Could you check a few things on this model? Use its own coordinates, in mm. A direction names the side the tool comes from. Coordinates: 2 decimals unless noted, no trailing zeros. Write each loop counter-clockwise with the first axis right and the second up, starting at its lowest first coordinate (ties: lowest second). Pieces come first, ordered by that corner, then holes.
Item 1: Which directions (+Z, -Z, +X, -X, +Y, -Y) give clear straight access to the entire face, cutting with the end or side of a thin tool? Please do faces 4 (the cylindrical face through (-16.52, -108.6, 7.96)), 5 (the flat face through (-18, 69, 7)), 6 (the flat face through (-25.2, 0.6, 13.75)), 7 (the flat face through (-18, -68, 7)).
Item 2: Thinking about a two-plate mould opening in Z: for faces 1 (the cylindrical face through (-16.52, 82.6, 7.96)), 2 (the flat face through (-22.4, 1.7, 15.75)), 3 (the cylindrical face through (-27, 0, 15)), which applies, +Z half, -Z half, draft (parallel to the pull), parting line (faces both ways), or undercut?
Item 3: I want a section at B-B on z = 2. Please give me the cut outline in (x, y).
Item 4: I want a section at C-C on y = -28. Please give me the cut outline in (x, z).
Item 5: If I drill on probe 1 along Z at (x, y) = (-16.75, -62.8) (3 decimals); probe 2 along X at (y, z) = (24, 11.5); probe 3 along Z at (x, y) = (-19, 22), over which ranges is the centre line in solid material (lowest first)?
Item 6: I want a section at D-D on y = 5. Please give me the cut outline in (x, z).
Item 7: For P1, Ø4.5, axis at y = 80.6, z = 7.875, coming from the -X side; P2, Ø3, axis at y = 32.8, z = 7.875, coming from the +X side; P3, Ø1, axis at y = -91, z = 14.5, coming from the -X side; P4, Ø2.5, axis at x = -21, y = 43.5, coming from the -Z side, each with a flat end and sliding along its axis, tell me the tip position at first contact or that it passes through.
Item 8: I want a section at A-A on y = 62.8. Please give me the cut outline in (x, z) (3 decimals), then the cut area to 4 significant figures.
from build123d import *

# Parameters (mm, degrees)
F1_DEPTH = 15.75
F2_R     = 2
F4_DEPTH = 3.001
F3_R     = 2
F5_DEPTH = 3.001
F7_DEPTH = 2


# Not quite as in the source:
# - a feature names something its author has since deleted; it is built from what else it names


with BuildPart() as f1:
    # F0 (on Top) → F1 (new body)
    with BuildSketch(Plane.XY):
        with BuildLine():
            Line((-15, 119.5), (-18, 119.5))
            Line((-18, 119.5), (-18, 17.3493515729))
            ThreePointArc((-18, 17.3493515729), (-25, 0), (-18, -17.3493515729))
            Line((-18, -17.3493515729), (-18, -119.5))
            Line((-18, -119.5), (-15, -119.5))
            Line((-15, -119.5), (-15, -16.0934769394))
            ThreePointArc((-15, -16.0934769394), (-16.5896327506, -14.4493627956), (-18, -12.6491106407))
            ThreePointArc((-18, -12.6491106407), (-22, 0), (-18, 12.6491106407))
            ThreePointArc((-18, 12.6491106407), (-16.5896327506, 14.4493627956), (-15, 16.0934769394))
            Line((-15, 16.0934769394), (-15, 119.5))
        make_face()
    extrude(amount=F1_DEPTH)

    # F2 (on face) → F4 (cut, through all)
    with BuildSketch(Plane(origin=(-18, 0, 0), x_dir=(0, -1, 0), z_dir=(-1, 0, 0))):
        with Locations((-110.6, 7.875)):
            Circle(F2_R)
        with Locations((-80.6, 7.875)):
            Circle(F2_R)
        with Locations((-62.8, 7.875)):
            Circle(F2_R)
        with Locations((-32.8, 7.875)):
            Circle(F2_R)
    extrude(amount=-F4_DEPTH, mode=Mode.SUBTRACT)

    # F3 (on face) → F5 (cut, through all)
    with BuildSketch(Plane(origin=(-18, 0, 0), x_dir=(0, -1, 0), z_dir=(-1, 0, 0))):
        with Locations((32.8, 7.875)):
            Circle(F3_R)
        with Locations((62.8, 7.875)):
            Circle(F3_R)
        with Locations((80.6, 7.875)):
            Circle(F3_R)
        with Locations((110.6, 7.875)):
            Circle(F3_R)
    extrude(amount=-F5_DEPTH, mode=Mode.SUBTRACT)

    # F6 (on face) → F7 (join)
    with BuildSketch(Plane.XY.offset(15.75)):
        with BuildLine():
            ThreePointArc((-20, 18.1383571472), (-27, 0), (-20, -18.1383571472))
            Line((-20, -18.1383571472), (-20, -119.5))
            Line((-20, -119.5), (-18, -119.5))
            Line((-18, -119.5), (-18, -17.3493515729))
            ThreePointArc((-18, -17.3493515729), (-25, 0), (-18, 17.3493515729))
            Line((-18, 17.3493515729), (-18, 119.5))
            Line((-18, 119.5), (-20, 119.5))
            Line((-20, 119.5), (-20, 18.1383571472))
        make_face()
    extrude(amount=-F7_DEPTH)


solid = f1.part
Response values:
1. face 4: +X, -X
1. face 5: -Z, -X, +Y
1. face 6: -Z, -X
1. face 7: -Z, -X, -Y
2. face 1: undercut
2. face 2: +Z half
2. face 3: draft
3. outline: (-18, -119.5) - (-15, -119.5) - (-15, -16.09) arc R22 cw to (-15, 16.09) - (-15, 119.5) - (-18, 119.5) - (-18, 17.35) arc R25 ccw to (-18, -17.35) - close
4. outline: (-20, 13.75) - (-18, 13.75) - (-18, 0) - (-15, 0) - (-15, 15.75) - (-20, 15.75) - close
5. probe 1: z = 0 to 5.875, 9.875 to 15.75
5. probe 2: x = -18 to -15
5. probe 3: z = 13.75 to 15.75
6. outline: (-26.53, 13.75) - (-24.49, 13.75) - (-24.49, 0) - (-21.42, 0) - (-21.42, 15.75) - (-26.53, 15.75) - close
7. P1: stops at x = -18
7. P2: passes through
7. P3: stops at x = -20
7. P4: stops at z = 13.75
8. outline: (-20, 13.75) - (-18, 13.75) - (-18, 9.875) - (-15, 9.875) - (-15, 15.75) - (-20, 15.75) - close; (-18, 0) - (-15, 0) - (-15, 5.875) - (-18, 5.875) - close
8. area: 39.25 mm2
